from build123d import *

# Parameters (mm, degrees)
BOSS_EXTRUDE1_DEPTH = 25
SKETCH4_R           = 6
CUT_EXTRUDE1_DEPTH  = 12
SKETCH5_R           = 3.2
CUT_EXTRUDE2_DEPTH  = 193.726734542
CHAMFER1_SIZE       = 0.5


with BuildPart() as part:
    # Sketch3 → Boss-Extrude1 (new body)
    with BuildSketch(Plane.XY):
        with BuildLine():
            Line((0, -25.695570819), (8.806669266, -122.712097135))
            ThreePointArc((8.806669266, -122.712097135), (18.452204227, -142.151330818), (38.683826579, -150))
            Line((38.683826579, -150), (81.316173421, -150))
            ThreePointArc((81.316173421, -150), (101.46473628, -142.226907448), (111.172189547, -122.935694313))
            Line((111.172189547, -122.935694313), (120.310407726, -30))
            ThreePointArc((120.310407726, -30), (111.523611161, -8.786796564), (90.310407726, 0))
            Line((90.310407726, 0), (29.689592274, 0))
            ThreePointArc((29.689592274, 0), (10.057130323, -7.315943094), (0, -25.695570819))
        make_face()
    extrude(amount=BOSS_EXTRUDE1_DEPTH)

    # Sketch4 → Cut-Extrude1 (cut)
    with BuildSketch(Plane.XY.offset(25)):
        with Locations((60, -34.5)):
            Circle(SKETCH4_R)
        with Locations((60, -112.5)):
            Circle(SKETCH4_R)
    extrude(amount=-CUT_EXTRUDE1_DEPTH, mode=Mode.SUBTRACT)

    # Sketch5 → Cut-Extrude2 (cut, through all)
    with BuildSketch(Plane.XY.offset(13)):
        with Locations((60, -34.5)):
            Circle(SKETCH5_R)
        with Locations((60, -112.5)):
            Circle(SKETCH5_R)
    extrude(amount=-CUT_EXTRUDE2_DEPTH, mode=Mode.SUBTRACT)

    # Chamfer1
    # the kernel refuses this chamfer: 0.5 mm, written as the material it takes off along each edge
    with BuildSketch(Plane(origin=(81.316173421, -120, 0), x_dir=(0, -1, 0), z_dir=(-1, 0, 0))) as chamfer1_piece_1:
        Polygon((30 - CHAMFER1_SIZE, 0), (30, CHAMFER1_SIZE), (30, 0), align=None)
    revolve(axis=Axis((81.316173421, -120, 0), (0, 0, 1)), revolution_arc=84.384249791, mode=Mode.SUBTRACT)
    with BuildSketch(Plane(origin=(38.683826579, -150, 0), x_dir=(0, 0.9996219169112968, -0.027495876610586483), z_dir=(1, 0, 0))) as chamfer1_piece_2:
        Polygon((CHAMFER1_SIZE * 0.999621916911, CHAMFER1_SIZE * 0.0274958766106), (-CHAMFER1_SIZE * 0.0274958766106, CHAMFER1_SIZE * 0.999621916911), (0, 0), align=None)
    extrude(amount=42.632346842, mode=Mode.SUBTRACT)
    with BuildSketch(Plane(origin=(38.683826579, -120, 0), x_dir=(-0.9959052437808521, -0.09040323782808642, 0), z_dir=(-0.09040323782808642, 0.9959052437808521, 0))) as chamfer1_piece_3:
        Polygon((30, CHAMFER1_SIZE), (30 - CHAMFER1_SIZE, 0), (30, 0), align=None)
    revolve(axis=Axis((38.683826579, -120, 0), (0, 0, 1)), revolution_arc=84.813194516, mode=Mode.SUBTRACT)
    with BuildSketch(Plane(origin=(-0.116244234, -24.414994532, 0), x_dir=(-0.027383287698834344, -0.0024857162725187313, 0.9996219169112968), z_dir=(0.09040323782809233, -0.9959052437808515, 0))) as chamfer1_piece_4:
        Polygon((CHAMFER1_SIZE * 0.999621916911, -CHAMFER1_SIZE * 0.0274958766106), (-CHAMFER1_SIZE * 0.0274958766106, -CHAMFER1_SIZE * 0.999621916911), (0, 0), align=None)
    extrude(amount=98.701260202, mode=Mode.SUBTRACT)
    with BuildSketch(Plane(origin=(38.683826579, -150, 25), x_dir=(0, 0.9996219169112968, 0.027495876610589196), z_dir=(1, 0, 0))) as chamfer1_piece_5:
        Polygon((CHAMFER1_SIZE * 0.999621916911, -CHAMFER1_SIZE * 0.0274958766106), (-CHAMFER1_SIZE * 0.0274958766106, -CHAMFER1_SIZE * 0.999621916911), (0, 0), align=None)
    extrude(amount=42.632346842, mode=Mode.SUBTRACT)
    with BuildSketch(Plane(origin=(81.316173421, -120, 25), x_dir=(0, -1, 0), z_dir=(-1, 0, 0))) as chamfer1_piece_6:
        Polygon((30 - CHAMFER1_SIZE, 0), (30, -CHAMFER1_SIZE), (30, 0), align=None)
    revolve(axis=Axis((81.316173421, -120, 25), (0, 0, 1)), revolution_arc=84.384249791, mode=Mode.SUBTRACT)
    with BuildSketch(Plane(origin=(111.172189547, -122.935694313, 25), x_dir=(-0.9948242690303891, 0.09781947923377807, 0.027495876610589255), z_dir=(0.09785647711289452, 0.9952005375234951, 0))) as chamfer1_piece_7:
        Polygon((CHAMFER1_SIZE * 0.999621916911, -CHAMFER1_SIZE * 0.0274958766106), (-CHAMFER1_SIZE * 0.0274958766106, -CHAMFER1_SIZE * 0.999621916911), (0, 0), align=None)
    extrude(amount=94.669728268, mode=Mode.SUBTRACT)
    with BuildSketch(Plane(origin=(90.310407726, -30, 25), x_dir=(0.9990808536319631, -0.04286546285796977, 0), z_dir=(-0.04286546285796977, -0.9990808536319631, 0))) as chamfer1_piece_8:
        Polygon((30 - CHAMFER1_SIZE, 0), (30, -CHAMFER1_SIZE), (30, 0), align=None)
    revolve(axis=Axis((90.310407726, -30, 25), (0, 0, 1)), revolution_arc=92.456762863, mode=Mode.SUBTRACT)
    with BuildSketch(Plane(origin=(60, -34.5, 25), x_dir=(1, 0, 0), z_dir=(0, -1, 0))) as chamfer1_piece_9:
        Polygon((6 + CHAMFER1_SIZE, 0), (6, -CHAMFER1_SIZE), (6, 0), align=None)
    revolve(axis=Axis((60, -34.5, 25), (0, 0, 1)), mode=Mode.SUBTRACT)
    with BuildSketch(Plane(origin=(90.310407726, 0, 25), x_dir=(0, -0.9996219169112968, 0.027495876610589425), z_dir=(-1, 0, 0))) as chamfer1_piece_10:
        Polygon((CHAMFER1_SIZE * 0.999621916911, -CHAMFER1_SIZE * 0.0274958766106), (-CHAMFER1_SIZE * 0.0274958766106, -CHAMFER1_SIZE * 0.999621916911), (0, 0), align=None)
    extrude(amount=60.620815451, mode=Mode.SUBTRACT)
    with BuildSketch(Plane(origin=(60, -112.5, 25), x_dir=(1, 0, 0), z_dir=(0, -1, 0))) as chamfer1_piece_11:
        Polygon((6 + CHAMFER1_SIZE, 0), (6, -CHAMFER1_SIZE), (6, 0), align=None)
    revolve(axis=Axis((60, -112.5, 25), (0, 0, 1)), mode=Mode.SUBTRACT)
    with BuildSketch(Plane(origin=(29.689592274, -30, 25), x_dir=(0, 1, 0), z_dir=(1, 0, 0))) as chamfer1_piece_12:
        Polygon((30, -CHAMFER1_SIZE), (30 - CHAMFER1_SIZE, 0), (30, 0), align=None)
    revolve(axis=Axis((29.689592274, -30, 25), (0, 0, 1)), revolution_arc=84.2072647, mode=Mode.SUBTRACT)
    with BuildSketch(Plane(origin=(60, -34.5, 0), x_dir=(1, 0, 0), z_dir=(0, -1, 0))) as chamfer1_piece_13:
        Polygon((3.2 + CHAMFER1_SIZE, 0), (3.2, CHAMFER1_SIZE), (3.2, 0), align=None)
    revolve(axis=Axis((60, -34.5, 0), (0, 0, 1)), mode=Mode.SUBTRACT)
    with BuildSketch(Plane(origin=(60, -112.5, 0), x_dir=(1, 0, 0), z_dir=(0, -1, 0))) as chamfer1_piece_14:
        Polygon((3.2 + CHAMFER1_SIZE, 0), (3.2, CHAMFER1_SIZE), (3.2, 0), align=None)
    revolve(axis=Axis((60, -112.5, 0), (0, 0, 1)), mode=Mode.SUBTRACT)
    with BuildSketch(Plane(origin=(-0.116244234, -24.414994532, 25), x_dir=(-0.027383287698834274, -0.002485716272518725, -0.9996219169112968), z_dir=(0.09040323782809233, -0.9959052437808515, 0))) as chamfer1_piece_15:
        Polygon((CHAMFER1_SIZE * 0.999621916911, CHAMFER1_SIZE * 0.0274958766106), (-CHAMFER1_SIZE * 0.0274958766106, CHAMFER1_SIZE * 0.999621916911), (0, 0), align=None)
    extrude(amount=98.701260202, mode=Mode.SUBTRACT)
    with BuildSketch(Plane(origin=(29.689592274, -30, 0), x_dir=(0, 1, 0), z_dir=(1, 0, 0))) as chamfer1_piece_16:
        Polygon((30, CHAMFER1_SIZE), (30 - CHAMFER1_SIZE, 0), (30, 0), align=None)
    revolve(axis=Axis((29.689592274, -30, 0), (0, 0, 1)), revolution_arc=84.2072647, mode=Mode.SUBTRACT)
    with BuildSketch(Plane(origin=(38.683826579, -120, 25), x_dir=(-0.9959052437808521, -0.09040323782808642, 0), z_dir=(-0.09040323782808642, 0.9959052437808521, 0))) as chamfer1_piece_17:
        Polygon((30, -CHAMFER1_SIZE), (30 - CHAMFER1_SIZE, 0), (30, 0), align=None)
    revolve(axis=Axis((38.683826579, -120, 25), (0, 0, 1)), revolution_arc=84.813194516, mode=Mode.SUBTRACT)
    with BuildSketch(Plane(origin=(90.310407726, 0, 0), x_dir=(0, -0.9996219169112968, -0.027495876610586893), z_dir=(-1, 0, 0))) as chamfer1_piece_18:
        Polygon((CHAMFER1_SIZE * 0.999621916911, CHAMFER1_SIZE * 0.0274958766106), (-CHAMFER1_SIZE * 0.0274958766106, CHAMFER1_SIZE * 0.999621916911), (0, 0), align=None)
    extrude(amount=60.620815451, mode=Mode.SUBTRACT)
    with BuildSketch(Plane(origin=(90.310407726, -30, 0), x_dir=(0.9990808536319631, -0.04286546285796977, 0), z_dir=(-0.04286546285796977, -0.9990808536319631, 0))) as chamfer1_piece_19:
        Polygon((30 - CHAMFER1_SIZE, 0), (30, CHAMFER1_SIZE), (30, 0), align=None)
    revolve(axis=Axis((90.310407726, -30, 0), (0, 0, 1)), revolution_arc=92.456762863, mode=Mode.SUBTRACT)
    with BuildSketch(Plane(origin=(111.172189547, -122.935694313, 0), x_dir=(-0.9948242690303891, 0.09781947923377807, -0.02749587661058666), z_dir=(0.09785647711289452, 0.9952005375234951, 0))) as chamfer1_piece_20:
        Polygon((CHAMFER1_SIZE * 0.999621916911, CHAMFER1_SIZE * 0.0274958766106), (-CHAMFER1_SIZE * 0.0274958766106, CHAMFER1_SIZE * 0.999621916911), (0, 0), align=None)
    extrude(amount=94.669728268, mode=Mode.SUBTRACT)


solid = part.part
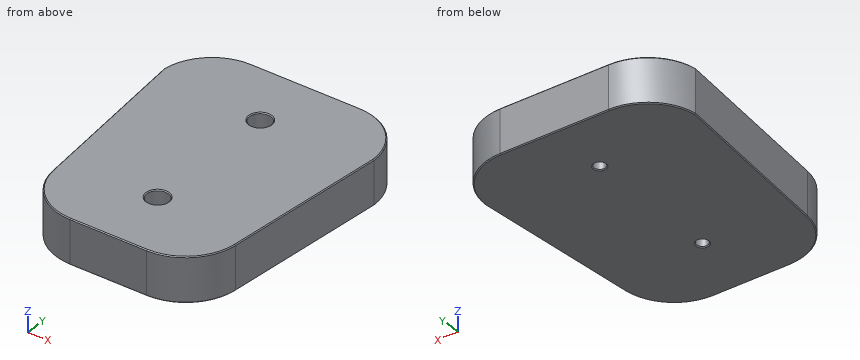
Verification items for the finished model (mm, model axes). Round coordinates to 2 decimals unless told otherwise and drop trailing zeros. Write each loop counter-clockwise with the first axis right and the second up, starting at its lowest first coordinate (ties: lowest second). Pieces come first, ordered by that corner, then holes.
(1) Depth check by flat-ended pin: pin 1 Ø5 at (y, z) = (-128, 9) entering from +X; pin 2 Ø3.5 at (x, y) = (62, -32) entering from +Z; pin 3 Ø3 at (x, z) = (102.5, 12) entering from -Y; pin 4 Ø4 at (x, y) = (60, -34.5) entering from -Z. Enter the tip coordinate at first touch or a pass-through.
Returned:
pin 1: stops at x = 110.81
pin 2: stops at z = 13
pin 3: stops at y = -142.64
pin 4: passes through
(2) Section check A-A (z = 4.25). Enter the section's corners in (x, y), plus the area to 3 significant figures.
Returned:
outline: (0, -25.7) - (8.81, -122.71) arc R30 ccw to (38.68, -150) - (81.32, -150) arc R30 ccw to (111.17, -122.94) - (120.31, -30) arc R30 ccw to (90.31, 0) - (29.69, 0) arc R30 ccw to start; hole circle Ø6.4 at (60, -112.5); hole circle Ø6.4 at (60, -34.5)
area: 15,900 mm2
(3) Material ranges on line 1 (Y direction, x = 60, z = 6.75); line 2 (Y direction, x = 60, z = 21.75); line 3 (X direction, y = -30, z = 2), recorded low to high.
Returned:
line 1: y = -150 to -115.7, -109.3 to -37.7, -31.3 to 0
line 2: y = -150 to -118.5, -106.5 to -40.5, -28.5 to 0
line 3: x = 0.39 to 120.31
(4) Section check C-C (y = -112.5). Enter the section's corners in (x, z).
Returned:
outline: (7.88, 0.5) - (8.38, 0) - (56.3, 0) - (56.8, 0.5) - (56.8, 13) - (54, 13) - (54, 24.5) - (53.5, 25) - (8.38, 25) - (7.88, 24.5) - close; (63.2, 0.5) - (63.7, 0) - (111.7, 0) - (112.2, 0.5) - (112.2, 24.5) - (111.7, 25) - (66.5, 25) - (66, 24.5) - (66, 13) - (63.2, 13) - close
(5) Section check D-D (z = 16). Enter the section's corners in (x, y).
Returned:
outline: (0, -25.7) - (8.81, -122.71) arc R30 ccw to (38.68, -150) - (81.32, -150) arc R30 ccw to (111.17, -122.94) - (120.31, -30) arc R30 ccw to (90.31, 0) - (29.69, 0) arc R30 ccw to start; hole circle Ø12 at (60, -112.5); hole circle Ø12 at (60, -34.5)
(6) Section check B-B (x = 60). Give the number of separate pieces and of enclosed holes in the cut face, plus the area to 3 significant figures.
Returned:
separate pieces: 3
enclosed holes: 0
area: 3,290 mm2
